Could you check a few things on this model? Use its own coordinates, in mm. Coordinates: 2 decimals unless noted, no trailing zeros. Loops run counter-clockwise (first coordinate to the right, second up) from the corner with the lowest first, then second, coordinate; pieces in that order, holes last.
from build123d import *

# Parameters (mm, degrees)
F0_W     = 1100
F0_H     = 1100
F1_DEPTH = 12
F2_R     = 7
F3_DEPTH = 25
F5_DEPTH = 25


# Not quite as in the source:
# - a feature names something its author has since deleted; it is built from what else it names


with BuildPart() as f1:
    # F0 (on Top) → F1 (new body)
    with BuildSketch(Plane.XY):
        Rectangle(F0_W, F0_H)
    extrude(amount=-F1_DEPTH)

    # F2 (on Top) → F3 (cut)
    with BuildSketch(Plane.XY):
        with Locations((-505, -505)):
            Circle(F2_R)
        with Locations((505, 505)):
            Circle(F2_R)
        with Locations((-505, 505)):
            Circle(F2_R)
        with Locations((505, -505)):
            Circle(F2_R)
    extrude(amount=-F3_DEPTH, mode=Mode.SUBTRACT)

    # F4 (on Top) → F5 (cut)
    with BuildSketch(Plane.XY):
        with BuildLine():
            Line((-80, 475), (-470, 475))
            ThreePointArc((-470, 475), (-473.5355339059, 473.5355339059), (-475, 470))
            Line((-475, 470), (-475, 80))
            ThreePointArc((-475, 80), (-473.5355339059, 76.4644660941), (-470, 75))
            Line((-470, 75), (-80, 75))
            ThreePointArc((-80, 75), (-76.4644660941, 76.4644660941), (-75, 80))
            Line((-75, 80), (-75, 470))
            ThreePointArc((-75, 470), (-76.4644660941, 473.5355339059), (-80, 475))
        make_face()
        with BuildLine():
            ThreePointArc((80, 475), (76.4644660941, 473.5355339059), (75, 470))
            Line((75, 470), (75, 80))
            ThreePointArc((75, 80), (76.4644660941, 76.4644660941), (80, 75))
            Line((80, 75), (470, 75))
            ThreePointArc((470, 75), (473.5355339059, 76.4644660941), (475, 80))
            Line((475, 80), (475, 470))
            ThreePointArc((475, 470), (473.5355339059, 473.5355339059), (470, 475))
            Line((470, 475), (80, 475))
        make_face()
        with BuildLine():
            ThreePointArc((475, -80), (473.5355339059, -76.4644660941), (470, -75))
            Line((470, -75), (80, -75))
            ThreePointArc((80, -75), (76.4644660941, -76.4644660941), (75, -80))
            Line((75, -80), (75, -470))
            ThreePointArc((75, -470), (76.4644660941, -473.5355339059), (80, -475))
            Line((80, -475), (470, -475))
            ThreePointArc((470, -475), (473.5355339059, -473.5355339059), (475, -470))
            Line((475, -470), (475, -80))
        make_face()
        with BuildLine():
            ThreePointArc((-475, -470), (-473.5355339059, -473.5355339059), (-470, -475))
            Line((-470, -475), (-80, -475))
            ThreePointArc((-80, -475), (-76.4644660941, -473.5355339059), (-75, -470))
            Line((-75, -470), (-75, -80))
            ThreePointArc((-75, -80), (-76.4644660941, -76.4644660941), (-80, -75))
            Line((-80, -75), (-470, -75))
            ThreePointArc((-470, -75), (-473.5355339059, -76.4644660941), (-475, -80))
            Line((-475, -80), (-475, -470))
        make_face()
    extrude(amount=-F5_DEPTH, mode=Mode.SUBTRACT)


solid = f1.part
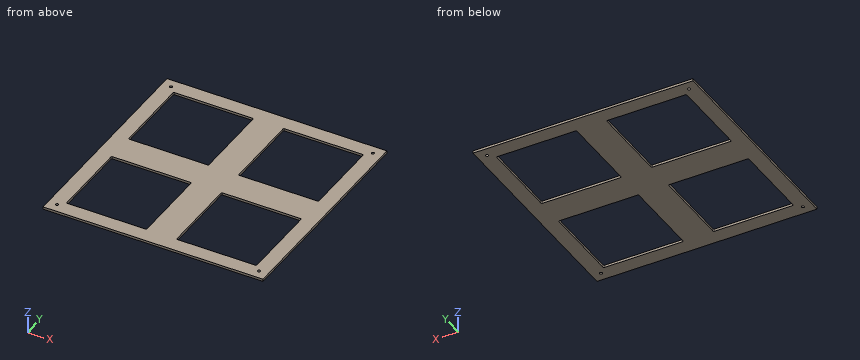
(1) I need wall thicknesses on probe 1 along Y at (x, z) = (-505, -6.75); probe 2 along X at (y, z) = (305, -1.25). Which ranges of each line are inside material? Lowest first, please.
Answers:
probe 1: y = -550 to -512, -498 to 498, 512 to 550
probe 2: x = -550 to -475, -75 to 75, 475 to 550
(2) For pin 1 (8.5 mm diameter, centred on x = -505, y = 505, fed in from +Z), with a flat end and sliding along its axis, tell me the tip position at first contact or that it passes through.
Answers:
pin 1: passes through
(3) Imagine slicing it at A-A, the plane y = 132. Write out the boundary of the cut face in (x, z).
Answers:
outline: (-550, -12) - (-475, -12) - (-475, 0) - (-550, 0) - close; (-75, -12) - (75, -12) - (75, 0) - (-75, 0) - close; (475, -12) - (550, -12) - (550, 0) - (475, 0) - close
(4) Imagine slicing it at C-C, the plane z = -6. State how many separate pieces and enclosed holes the cut face has, and give its area (3 significant figures).
Answers:
separate pieces: 1
enclosed holes: 8
area: 569,000 mm2
